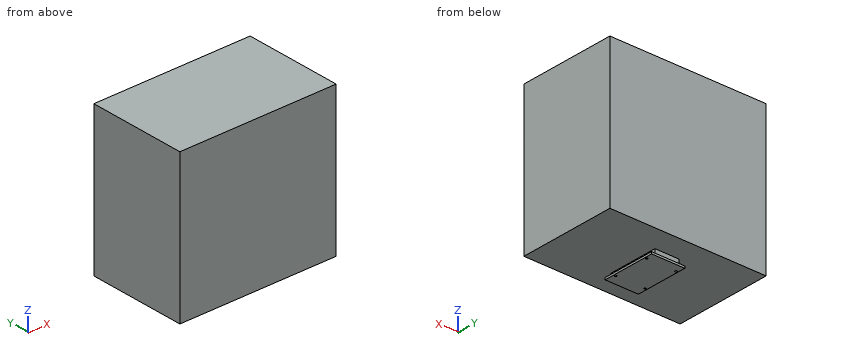
```python
from build123d import *

# Parameters (mm, degrees)
F0_W     = 215.9
F0_H     = 342.9
F0_R     = 6.35
F1_DEPTH = 12.7
F2_W     = 155.575
F2_H     = 323.85
F3_DEPTH = 44.45
F4_W     = 1016
F4_H     = 635
F5_DEPTH = 965.2


with BuildPart() as f1:
    # F0 (on Top) → F1 (new body)
    with BuildSketch(Plane.XY):
        Rectangle(F0_W, F0_H)
        with Locations((-95.25, -107.95)):
            Circle(F0_R, mode=Mode.SUBTRACT)
        with Locations((95.25, -107.95)):
            Circle(F0_R, mode=Mode.SUBTRACT)
        with Locations((-95.25, 120.65)):
            Circle(F0_R, mode=Mode.SUBTRACT)
        with Locations((95.25, 120.65)):
            Circle(F0_R, mode=Mode.SUBTRACT)
    extrude(amount=F1_DEPTH)

    # F2 (on face) → F3 (join)
    with BuildSketch(Plane.XY):
        Rectangle(F2_W, F2_H)
    extrude(amount=F3_DEPTH)

    # F4 (on face) → F5 (join)
    with BuildSketch(Plane.XY.offset(44.45)):
        Rectangle(F4_W, F4_H)
    extrude(amount=F5_DEPTH)


solid = f1.part
```
Check sheet for the modelled part. Datum: model origin and axes. Units: mm. Give positions to 0.01 mm unless a question says otherwise; leave off trailing zeros. Order: outer loops, then holes, each group sorted by start corner. A loop starts at its lowest first (then second) coordinate and runs counter-clockwise, first axis right, second up. Notation, with made-up numbers: (-18, 27.5) -> (-4, 27.5) arc R10 cw to (-4, 39.5) -> close; hole circle Ø2 at (-37, -33.75). An arc over 180 degrees is marked (long way). Use CSV: the item, a comma, the result in double quotes. Start each with the question number.
1) Sectioned sample at C-C, the plane y = 228. Record the boundary of the cut face in (x, z).
2) Go/stop test with flat-tipped pins: P1, Ø16, axis at y = 75, z = 24.5, coming from the -X side; P2, Ø7.5, axis at x = -95.25, y = -107.95, coming from the -Z side; P3, Ø4, axis at y = -51.5, z = 7, coming from the -X side. Record where each tip stops, or that it passes through.
3) Sectioned sample at A-A, the plane y = -129.5. Record the boundary of the cut face in (x, z).
4) Sectioned sample at B-B, the plane x = -330. Record the boundary of the cut face in (y, z).
5) Material ranges on line 1 (Y direction, x = -95.25, z = 6.5); line 2 (X direction, y = -107, z = 2); line 3 (Z direction, x = 86, y = 110.5), recorded low to high. Write a range as from..to.
Recorded:
1,outline,"(-508, 44.45) -> (508, 44.45) -> (508, 1009.65) -> (-508, 1009.65) -> close"
2,P1,"x = -77.79"
2,P2,"z = 44.45"
2,P3,"x = -107.95"
3,outline,"(-508, 44.45) -> (-77.79, 44.45) -> (-77.79, 12.7) -> (-107.95, 12.7) -> (-107.95, 0) -> (107.95, 0) -> (107.95, 12.7) -> (77.79, 12.7) -> (77.79, 44.45) -> (508, 44.45) -> (508, 1009.65) -> (-508, 1009.65) -> close"
4,outline,"(-317.5, 44.45) -> (317.5, 44.45) -> (317.5, 1009.65) -> (-317.5, 1009.65) -> close"
5,line 1,"-171.45..-114.3, -101.6..114.3, 127..171.45"
5,line 2,"-107.95..-101.53, -88.97..88.97, 101.53..107.95"
5,line 3,"0..12.7, 44.45..1009.65"
